Check sheet for the modelled part. Datum: model origin and axes. Units: mm. A direction names the side the tool comes from. Give positions to 0.01 mm unless a question says otherwise; leave off trailing zeros. Order: outer loops, then holes, each group sorted by start corner. A loop starts at its lowest first (then second) coordinate and runs counter-clockwise, first axis right, second up.
Item 1: Sectioned sample at A-A on z = 7.25. Record the boundary of the cut face in (x, y).
Item 2: Sectioned sample at B-B on y = -2.5. Record the boundary of the cut face in (x, z).
Item 3: Gauge pin test, flat end, axial feed: P1, Ø4, axis at x = -15, y = -3, coming from the +Z side. Record the tip position at first contact, or that the pin passes through.
Item 4: Release check for a two-part mould opening along Y. For faces 1 (the flat face through (-32, 3, 12)), 2 (the flat face through (0, -5, 2)), 3 (the flat face through (30, -1.5, 7)) record: released by +Y, released by -Y, zero draft, split by the parting line, or undercut.
Item 5: Sectioned sample at C-C on x = 22. Record the boundary of the cut face in (y, z), and give its area (3 significant figures).
Item 6: Access from +Z, -Z, +X, -X, +Y, -Y to the whole of each face (thin tool, end or side, straight path). Record for faces 4 (the cylindrical face through (-26.641, -3.274, 10.797)), 5 (the flat face through (32, 3, 12)), 6 (the flat face through (-30, 1.5, 7)).
Item 7: Material ranges on line 1 along Y through (x, z) = (-30, 5.75); line 2 along X through (y, z) = (3, 8.25); line 3 along Z through (x, y) = (18, 0.75), recorded low to high.
from build123d import *

# Parameters (mm, degrees)
F2_W     = 69
F2_H     = 10
F3_DEPTH = 3
F4_W     = 9
F4_H     = 3.5
F5_DEPTH = 9
F6_R     = 4


with BuildPart() as f3:
    # F2 (on Top) → F3 (new body)
    with BuildSketch(Plane.XY):
        Rectangle(F2_W, F2_H)
    extrude(amount=F3_DEPTH)

    # F4 (on face) → F5 (join)
    with BuildSketch(Plane.XY.offset(3)):
        with Locations((-30, 3.25)):
            Rectangle(F4_W, F4_H)
    extrude(amount=F5_DEPTH)

    # F6
    f6_edges = [f3.edges().sort_by_distance(p)[0] for p in [
        (-25.5, 3.25, 12),
    ]]
    fillet(f6_edges, radius=F6_R)

    # F7: F3 across plane


with BuildPart() as f3_1:
    add(f3.part)
    add(f3.part.mirror(Plane.YZ))

    # F8: F3 across plane


with BuildPart() as f3_2:
    add(f3_1.part)
    add(f3_1.part.mirror(Plane.XZ))


solid = f3_2.part
Report:
1. outline: (-34.5, -5) - (-25.5, -5) - (-25.5, -1.5) - (-34.5, -1.5) - close; (-34.5, 1.5) - (-25.5, 1.5) - (-25.5, 5) - (-34.5, 5) - close; (25.5, -5) - (34.5, -5) - (34.5, -1.5) - (25.5, -1.5) - close; (25.5, 1.5) - (34.5, 1.5) - (34.5, 5) - (25.5, 5) - close
2. outline: (-34.5, 0) - (34.5, 0) - (34.5, 12) - (29.5, 12) arc R4 ccw to (25.5, 8) - (25.5, 3) - (-25.5, 3) - (-25.5, 8) arc R4 ccw to (-29.5, 12) - (-34.5, 12) - close
3. P1: stops at z = 3
4. face 1: zero draft
4. face 2: released by -Y
4. face 3: undercut
5. outline: (-5, 0) - (5, 0) - (5, 3) - (-5, 3) - close
5. area: 30.0 mm2
6. face 4: +Z, +Y, -Y
6. face 5: +Z, +X, -X, +Y, -Y
6. face 6: +Z, +X, -X
7. line 1: y = -5 to -1.5, 1.5 to 5
7. line 2: x = -34.5 to -25.51, 25.51 to 34.5
7. line 3: z = 0 to 3
